The listing builds one solid part. Answer for the finished solid, in the listing's coordinates (mm). A direction names the side the tool comes from. Give positions to 0.01 mm unless a question says otherwise; leave off trailing zeros. Write each loop counter-clockwise with the first axis right and the second up, starting at its lowest first coordinate (ties: lowest second). Pieces come first, ordered by that corner, then holes. Notation, with made-up numbers: (84, 64.25) - (124, 64.25) arc R34 cw to (124, 102.25) - close; hole circle Ø6 at (72, 84.5). An arc over 180 degrees is marked (long way). Answer in a Markdown table with one row per item. Add a question column.
from build123d import *

# Parameters (mm, degrees)
F0_R      = 20
F1_DEPTH  = 50
F2_DEPTH  = 30
F3_W      = 32
F3_H      = 52
F4_DEPTH  = 988.001
F5_W      = 30
F5_H      = 40
F5_W_2    = 24
F5_H_2    = 34
F6_DEPTH  = 350
F8_DEPTH  = 700
F9_DEPTH  = 200
F10_W     = 27.8917610645
F10_H     = 30
F10_W_2   = 29.6796619892
F10_W_3   = 29.7341316938
F10_W_4   = 29.711586237
F11_DEPTH = 25
F12_W     = 50
F12_H     = 50
F13_DEPTH = 10
F14_W     = 50
F14_H     = 50
F14_W_2   = 42
F14_H_2   = 42
F15_DEPTH = 600
F16_R     = 7.5
F16_R_2   = 5.5
F17_DEPTH = 20.5


# Not quite as in the source:
# - the program builds the solid bodies; features that only make, move or delete a surface that nothing else refers to are left out


with BuildPart() as f1:
    # F0 (on Front) → F1 (new body, symmetric)
    with BuildSketch(Plane.XZ):
        with BuildLine():
            ThreePointArc((20, -15), (23.7170824513, -7.9056941504), (25, 0))
            ThreePointArc((25, 0), (-7.9056941504, 23.7170824513), (-20, -15))
            ThreePointArc((-20, -15), (0, -25), (20, -15))
        make_face()
        Circle(F0_R, mode=Mode.SUBTRACT)
    extrude(amount=F1_DEPTH, both=True)

    # F0 (on Front) → F2 (join, symmetric)
    with BuildSketch(Plane.XZ):
        with BuildLine():
            ThreePointArc((20, -15), (0, -25), (-20, -15))
            Line((-20, -15), (-20, -1000))
            Line((-20, -1000), (20, -1000))
            Line((20, -1000), (20, -15))
        make_face()
    extrude(amount=F2_DEPTH, both=True)

    # F3 (on face) → F4 (cut, through all)
    with BuildSketch(Plane(origin=(0, 0, -1000), x_dir=(1, 0, 0), z_dir=(0, 0, -1))):
        Rectangle(F3_W, F3_H)
    extrude(amount=-F4_DEPTH, mode=Mode.SUBTRACT)

    # F5 (on Right) → F6 (join, symmetric)
    with BuildSketch(Plane.YZ):
        with Locations((15, -1020)):
            Rectangle(F5_W, F5_H)
        with Locations((15, -1020)):
            Rectangle(F5_W_2, F5_H_2, mode=Mode.SUBTRACT)
    extrude(amount=F6_DEPTH, both=True)

    # F7 (on face) → F8 (join)
    with BuildSketch(Plane.XZ):
        Polygon((-16, -1000), (-20, -1000), (-20, -1020), (-20, -1040), (20, -1040), (20, -1000), (16, -1000), align=None)
        Polygon((-17, -1037), (-17, -1020), (-17, -1003), (17, -1003), (17, -1037), align=None, mode=Mode.SUBTRACT)
    extrude(amount=F8_DEPTH)

    # F5 (on Right) → F9 (join, symmetric)
    with BuildSketch(Plane.YZ):
        with Locations((-715, -1020)):
            Rectangle(F5_W, F5_H)
        with Locations((-715, -1020)):
            Rectangle(F5_W_2, F5_H_2, mode=Mode.SUBTRACT)
    extrude(amount=F9_DEPTH, both=True)

    # F10 (on face) → F11 (join)
    with BuildSketch(Plane(origin=(0, 0, -1040), x_dir=(1, 0, 0), z_dir=(0, 0, -1))):
        with Locations((-336.0541194677, -15)):
            Rectangle(F10_W, F10_H)
        with Locations((335.1601690054, -15)):
            Rectangle(F10_W_2, F10_H)
        with Locations((-185.1329341531, 715)):
            Rectangle(F10_W_3, F10_H)
        with Locations((185.1442068815, 715)):
            Rectangle(F10_W_4, F10_H)
    extrude(amount=F11_DEPTH)

    # F12 (on face) → F13 (join)
    with BuildSketch(Plane.XZ.offset(50)):
        Rectangle(F12_W, F12_H)
    extrude(amount=F13_DEPTH)

    # F14 (on face) → F15 (join)
    with BuildSketch(Plane.XZ.offset(60)):
        Rectangle(F14_W, F14_H)
        Rectangle(F14_W_2, F14_H_2, mode=Mode.SUBTRACT)
    extrude(amount=F15_DEPTH)

    # F16 (on Right) → F17 (join, symmetric)
    with BuildSketch(Plane.YZ):
        with Locations((0, -840)):
            Circle(F16_R)
        with Locations((0, -840)):
            Circle(F16_R_2, mode=Mode.SUBTRACT)
    extrude(amount=F17_DEPTH, both=True)


solid = f1.part
1. A tool of negligible diameter and unlimited length cuts with its end or side. For faces 1 (the face through (0, -356, 21)), 2 (the face through (17, -345, -1020)), 3 (the face through (3, -715, -1037)), 4 (the face through (-322.108, 15, -1052)), from which of +Z, -Z, +X, -X, +Y, -Y can it reach the whole face along a straight path? Write none if from no direction.
2. Section A-A (y = -431.5) is taken. Give the vertices of the cut face in (x, z), and give its area (3 significant figures).
3. Given pin 1 Ø21 at (y, z) = (-474, 6.5) entering from -X; pin 2 Ø20 at (x, z) = (-1, -7.5) entering from +Y; pin 3 Ø17 at (x, y) = (-5, -480.5) entering from -Z, each flat-ended and moving along its own axis, determine where each tip first touches the part or whether it passes through.
4. Section B-B (x = 151.5) is taken. Give the vertices of the cut face in (y, z).
5. Section D-D (x = -233) is taken. Give the vertices of the cut face in (y, z).
6. Straight lines are drawn through the part: L1, parallel to Z at x = -14, y = -435; L2, parallel to Y at x = -8, z = -840; L3, parallel to Z at x = 0, y = -11. For each, find the intervals that lie inside material, in ascending order. Write a range as [from, to].
7. Section C-C (z = -879) is taken. Give the vertices of the cut face in (x, y), and give its area (3 significant figures).
8. The mould has two halves that part along Z. Classify faces 5 (the face through (-170.266, -715, -1052)), 6 (the face through (20, -9, -682)), 7 (the face through (-336, 15, -1065)): +Z half, -Z half, draft (parallel to the pull), parting line (faces both ways), or undercut.
Geometry check:
| question | item | result |
|---|---|---|
| 1 | face 1 | -Y |
| 1 | face 2 | none |
| 1 | face 3 | +X, -X |
| 1 | face 4 | -Z, +Y, -Y |
| 2 | outline | (-25, -25) - (25, -25) - (25, 25) - (-25, 25) - close; (-20, -1040) - (20, -1040) - (20, -1000) - (-20, -1000) - close; hole (-21, -21) - (21, -21) - (21, 21) - (-21, 21) - close; hole (-17, -1037) - (17, -1037) - (17, -1003) - (-17, -1003) - close |
| 2 | area | 1,180 mm² |
| 3 | pin 1 | x = -25 |
| 3 | pin 2 | y = -50 |
| 3 | pin 3 | z = -1040 |
| 4 | outline | (-730, -1040) - (-700, -1040) - (-700, -1000) - (-730, -1000) - close; (0, -1040) - (30, -1040) - (30, -1000) - (0, -1000) - close; hole (-727, -1037) - (-703, -1037) - (-703, -1003) - (-727, -1003) - close; hole (3, -1037) - (27, -1037) - (27, -1003) - (3, -1003) - close |
| 5 | outline | (0, -1040) - (30, -1040) - (30, -1000) - (0, -1000) - close; hole (3, -1037) - (27, -1037) - (27, -1003) - (3, -1003) - close |
| 6 | L1 | [-1040, -1037], [-1003, -1000], [-25, -21], [21, 25] |
| 6 | L2 | [-30, -26], [-7.5, -5.5], [5.5, 7.5], [26, 30] |
| 6 | L3 | [-1040, -1037], [-1003, -1000], [20, 25] |
| 7 | outline | (-20, -30) - (20, -30) - (20, 30) - (-20, 30) - close; hole (-16, -26) - (16, -26) - (16, 26) - (-16, 26) - close |
| 7 | area | 736 mm² |
| 8 | face 5 | draft |
| 8 | face 6 | undercut |
| 8 | face 7 | -Z half |
